```python
from build123d import *

# Parameters (mm, degrees)
F0_W      = 70
F0_H      = 20
F1_DEPTH  = 3
F3_DEPTH  = 9
F5_DEPTH  = 25
F6_R      = 1
F7_DEPTH  = 25
F8_R      = 2.5
F9_DEPTH  = 25
F10_W     = 3
F10_H     = 3
F11_DEPTH = 12
F12_SIZE  = 2.99999


# Not quite as in the source:
# - a fillet or chamfer is up to 0.001 mm smaller than in the source, because OpenCascade refuses the exact size


with BuildPart() as f1:
    # F0 (on Right) → F1 (new body)
    with BuildSketch(Plane.YZ):
        with Locations((15.2043993567, 29.5881517231)):
            Rectangle(F0_W, F0_H)
    extrude(amount=F1_DEPTH)

    # F2 (on face) → F3 (join)
    with BuildSketch(Plane.YZ.offset(3)):
        with BuildLine():
            ThreePointArc((-1.3103192691, 22.5881517231), (-3.0917046048, 20.8670406755), (-5.2130249484, 19.5881517231))
            Line((-5.2130249484, 19.5881517231), (0.2043993567, 19.5881517231))
            Line((0.2043993567, 19.5881517231), (0.2043993567, 22.5881517231))
            Line((0.2043993567, 22.5881517231), (-1.3103192691, 22.5881517231))
        make_face()
        with BuildLine():
            Line((0.2043993567, 22.5881517231), (0.2043993567, 19.5881517231))
            Line((0.2043993567, 19.5881517231), (35.6218236617, 19.5881517231))
            ThreePointArc((35.6218236617, 19.5881517231), (33.5005033181, 20.8670406755), (31.7191179824, 22.5881517231))
            Line((31.7191179824, 22.5881517231), (0.2043993567, 22.5881517231))
        make_face()
    extrude(amount=F3_DEPTH)

    # F4 (on face) → F5 (cut)
    with BuildSketch(Plane(origin=(0, 0, 0), x_dir=(0, -1, 0), z_dir=(-1, 0, 0))):
        with BuildLine():
            Line((19.7956006433, 29.5881517231), (19.7956006433, 39.5881517231))
            Line((19.7956006433, 39.5881517231), (9.7956006433, 39.5881517231))
            ThreePointArc((9.7956006433, 39.5881517231), (16.8666684552, 36.659219535), (19.7956006433, 29.5881517231))
        make_face()
        with BuildLine():
            Line((19.7956006433, 19.5881517231), (19.7956006433, 29.5881517231))
            ThreePointArc((19.7956006433, 29.5881517231), (16.8666684552, 22.5170839113), (9.7956006433, 19.5881517231))
            Line((9.7956006433, 19.5881517231), (19.7956006433, 19.5881517231))
        make_face()
        with BuildLine():
            ThreePointArc((-50.2043993567, 29.5881517231), (-47.2754671685, 36.659219535), (-40.2043993567, 39.5881517231))
            Line((-40.2043993567, 39.5881517231), (-50.2043993567, 39.5881517231))
            Line((-50.2043993567, 39.5881517231), (-50.2043993567, 29.5881517231))
        make_face()
        with BuildLine():
            ThreePointArc((-40.2043993567, 19.5881517231), (-47.2754671685, 22.5170839113), (-50.2043993567, 29.5881517231))
            Line((-50.2043993567, 29.5881517231), (-50.2043993567, 19.5881517231))
            Line((-50.2043993567, 19.5881517231), (-40.2043993567, 19.5881517231))
        make_face()
    extrude(amount=-F5_DEPTH, mode=Mode.SUBTRACT)

    # F6 (on face) → F7 (cut)
    with BuildSketch(Plane.YZ.offset(3)):
        with Locations((-9.7956006433, 29.5881517231)):
            Circle(F6_R)
        with Locations((40.2043993567, 29.5881517231)):
            Circle(F6_R)
    extrude(amount=-F7_DEPTH, mode=Mode.SUBTRACT)

    # F8 (on face) → F9 (cut)
    with BuildSketch(Plane(origin=(0, 0, 0), x_dir=(0, -1, 0), z_dir=(-1, 0, 0))):
        with Locations((-27.7043993567, 29.5881517231)):
            Circle(F8_R)
        with Locations((-15.2043993567, 29.5881517231)):
            Circle(F8_R)
    extrude(amount=-F9_DEPTH, mode=Mode.SUBTRACT)

    # F10 (on face) → F11 (join)
    with BuildSketch(Plane(origin=(0, 0, 0), x_dir=(0, -1, 0), z_dir=(-1, 0, 0))):
        Polygon((-8.2043993567, 16.5881517231), (-8.2043993567, 19.5881517231), (-33.2043993567, 19.5881517231), (-33.2043993567, 16.5881517231), (-15.2043993567, 16.5881517231), (-12.2043993567, 16.5881517231), align=None)
        with Locations((-13.7043993567, 15.0881517231)):
            Rectangle(F10_W, F10_H)
    extrude(amount=-F11_DEPTH)

    # F12 (size 3 in the source; OpenCascade refuses exactly that, so slightly less here)
    f12_edges = [f1.edges().sort_by_distance(p)[0] for p in [
        (6, 8.204399, 16.588152),
        (6, 33.204399, 16.588152),
    ]]
    chamfer(f12_edges, length=F12_SIZE)


solid = f1.part
```
Here's how the part is built. I have some questions about the finished solid (model axes, mm). A direction names the side the tool comes from. Give positions to 0.01 mm unless a question says otherwise; leave off trailing zeros. Write each loop counter-clockwise with the first axis right and the second up, starting at its lowest first coordinate (ties: lowest second). Pieces come first, ordered by that corner, then holes. Notation, with made-up numbers: (22.5, -36.5) -> (36.5, -36.5) arc R24 ccw to (36.5, -5.5) -> close; hole circle Ø5 at (47, -19.75). An arc over 180 degrees is marked (long way). Use one line per item in the form item = value.
1) Suppose I cut it at C-C (z = 21). Please give me the cut outline in (x, y).
Verdict:
outline = (0, -14.92) -> (3, -14.92) -> (3, -2.92) -> (12, -2.92) -> (12, 33.33) -> (3, 33.33) -> (3, 45.33) -> (0, 45.33) -> close
2) Suppose I cut it at A-A (x = 1.5). Give the number of separate pieces and of enclosed holes in the cut face, and give its area (3 significant figures).
Verdict:
separate_pieces = 1
enclosed_holes = 4
area = 1,340 mm2
3) I'm going to push flat-ended pins straight in: pin 1 (2 mm diameter, centred on x = 5, y = 36, fed in from -Z); pin 2 (1 mm diameter, centred on x = 2, z = 18.5, fed in from +Y); pin 3 (1.5 mm diameter, centred on x = 3.5, z = 23.5, fed in from -Y). Where does each tip first touch, or does it pass through?
Verdict:
pin_1 = 19.59
pin_2 = 32.62
pin_3 = -18.13
4) Suppose I cut it at D-D (y = 3.5). Please give me the cut outline in (x, z), and give its area (3 significant figures).
Verdict:
outline = (0, 19.59) -> (12, 19.59) -> (12, 22.59) -> (3, 22.59) -> (3, 39.59) -> (0, 39.59) -> close
area = 87.0 mm2
5) If I drill on L1, parallel to X at y = -4.5, z = 36.5; L2, parallel to Z at x = 7.75, y = 30; L3, parallel to Z at x = 3.5, y = -0.5, over which ranges is the centre line in solid material (lowest first)? Write a range as [from, to].
Verdict:
L1 = [0, 3]
L2 = [16.59, 22.59]
L3 = [19.59, 22.59]
6) On a 3-axis mill with a long thin cutter (end or side, diameter ignored), from which of +Z, -Z, +X, -X, +Y, -Y can I reach the whole of each face in a straight line? I mean faces 5 (the face through (6, 1, 19.588)), 6 (the face through (7.44, -3.06, 20.89)), 7 (the face through (6, 15.204, 15)), 8 (the face through (7, 15, 22.588)). Say none if no direction works.
Verdict:
face_5 = -Z, +X, -X, -Y
face_6 = +Z, +X, -Y
face_7 = -Z, +X, -X, +Y
face_8 = +Z, +X, +Y, -Y
7) We'd pull the mould along Y, two halves only. Please class faces 1 (the face through (12, 15, 20)), 2 (the face through (7.437, 33.528, 20.846)), 3 (the face through (1.479, 28.03, 32.067)), 4 (the face through (5.916, 9.725, 18.067)): +Y half, -Y half, draft (parallel to the pull), parting line (faces both ways), or undercut.
Verdict:
face_1 = draft
face_2 = +Y half
face_3 = undercut
face_4 = -Y half
